The model under review builds one solid part; all positions refer to its coordinate system, in mm. A direction names the side the tool comes from. Give positions to 0.01 mm unless a question says otherwise; leave off trailing zeros. Order: outer loops, then holes, each group sorted by start corner. A loop starts at its lowest first (then second) coordinate and runs counter-clockwise, first axis right, second up. Notation, with made-up numbers: (-34, 23.5) - (-1, 23.5) arc R18 cw to (-1, 57.5) - close; hole circle Ø9 at (6, 37.25). An arc over 180 degrees is marked (long way). Write item = value, one per line. Start each with the question number.
1. Mouldability with a two-part tool opening along Y and no side actions: class faces 1 (the flat face through (2, -5, 1)), 2 (the flat face through (2, -13, 1)), 3 (the flat face through (0.99, -16.61, -0.72)) as pulls with the +Y half, pulls with the -Y half, needs draft (parallel to the pull), parting line crosses it, or undercut.
2. We need section B-B, the plane z = 0.6. Give the boundary of the cut face in (x, y), and give its area (3 significant figures).
3. Wall thickness on probe 1 along Y at (x, z) = (3.5, 0.35); probe 2 along Z at (x, y) = (1.75, -13); probe 3 along X at (y, z) = (-5.25, 1.3): over which ranges is each line inside the solid? List them lowest first.
4. Machinability: for faces 4 (the flat face through (4, -9, 1)), 5 (the flat face through (5, -3, 1)), 6 (the flat face through (2.7, -7.4, 0)), 7 (the flat face through (3, -7, 1)), which of the approach directions +Z, -Z, +X, -X, +Y, -Y give a long, thin tool a straight path to every point of the face, cutting with its end or side? Answer none if there is none.
5. For P1, Ø2, axis at x = 1.5, z = 1.5, coming from the -Y side; P2, Ø1, axis at x = 5.5, z = 1, coming from the +Y side; P3, Ø1.9, axis at y = -12.5, z = 0.5, coming from the +X side, all flat-tipped, find the tip position at first contact; note any pin that passes through.
6. We need section D-D, the plane x = 3. Give the boundary of the cut face in (y, z), and give its area (3 significant figures).
7. We need section C-C, the plane y = -14.25. Give the boundary of the cut face in (x, z), and give its area (3 significant figures).
8. We need section A-A, the plane x = 0.5. Give the boundary of the cut face in (y, z), and give its area (3 significant figures).
from build123d import *

# Parameters (mm, degrees)
SKETCH_1_W      = 2
SKETCH_1_H      = 7.18
SKETCH_1_H_2    = 5
EXTRUDE_1_DEPTH = 2
EXTRUDE_2_DEPTH = 2


with BuildPart() as part:
    # 草图1 → 凸台-拉伸1 (new body)
    with BuildSketch(Plane.XY):
        with Locations((1, -12.59)):
            Rectangle(SKETCH_1_W, SKETCH_1_H)
        Polygon((5, -9), (5, -7), (0, -7), (0, -9), (2, -9), align=None)
        Polygon((7, -5), (5, -5), (5, -7), (5, -9), (7, -9), align=None)
        with Locations((1, -2.5)):
            Rectangle(SKETCH_1_W, SKETCH_1_H_2)
        Polygon((7, -3), (2, -3), (2, -5), (5, -5), (7, -5), align=None)
    extrude(amount=EXTRUDE_1_DEPTH)

    # 草图2 → 凸台-拉伸2 (add)
    with BuildSketch(Plane.ZY):
        Polygon((2, -16.18), (0.267949192, -17.18), (-1.732050808, -16.025299462), (0, -15.025299462), align=None)
    extrude(amount=-EXTRUDE_2_DEPTH)


solid = part.part
Model answer:
q1.face_1 = undercut
q1.face_2 = needs draft
q1.face_3 = pulls with the -Y half
q2.outline = (0, -16.99) - (2, -16.99) - (2, -9) - (7, -9) - (7, -3) - (2, -3) - (2, 0) - (0, 0) - (0, -5) - (5, -5) - (5, -7) - (0, -7) - close
q2.area = 54.0 mm2
q3.probe_1 = -9 to -7, -5 to -3
q3.probe_2 = 0 to 2
q3.probe_3 = 5 to 7
q4.face_4 = +Z, -Z, +X, -Y
q4.face_5 = +Z, -Z, +X, +Y
q4.face_6 = -Z, +X, -X, +Y
q4.face_7 = +Z, -Z, -X
q5.P1 = -17.05
q5.P2 = -3
q5.P3 = 2
q6.outline = (-9, 0) - (-7, 0) - (-7, 2) - (-9, 2) - close; (-5, 0) - (-3, 0) - (-3, 2) - (-5, 2) - close
q6.area = 8.00 mm2
q7.outline = (0, 0) - (2, 0) - (2, 2) - (0, 2) - close
q7.area = 4.00 mm2
q8.outline = (-17.18, 0.27) - (-16.03, -1.73) - (-15.03, 0) - (-7, 0) - (-7, 2) - (-16.18, 2) - close; (-5, 0) - (0, 0) - (0, 2) - (-5, 2) - close
q8.area = 31.2 mm2
